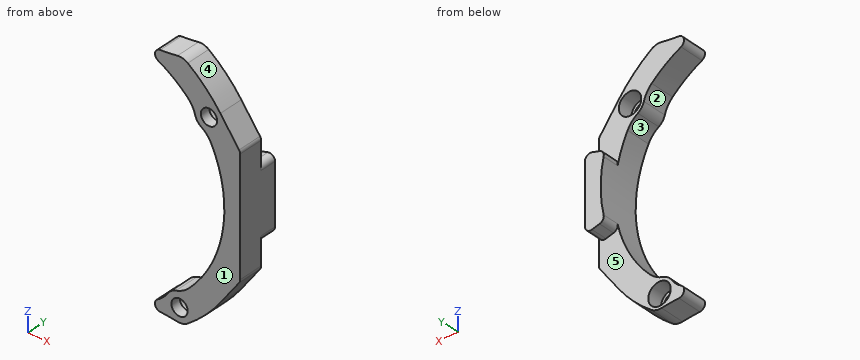
from build123d import *

# Parameters (mm, degrees)
SKETCH_1_R                     = 1.0250000000000292
EXTRUDE_1_DEPTH                = 4.5
EXTRUDE_1_2_DEPTH              = 4.5
EXTRUDE_START                  = -4.5
EXTRUDE_2_DEPTH                = 4.5
EXTRUDE_3_DEPTH                = 3
SKETCH_7_R                     = 1.45
SKETCH_7_R_2                   = 1.0000000000000018
EXTRUDE_5_DEPTH                = 4.5
HOLE_WIZARD_M2_5_2_D           = 2.9
HOLE_WIZARD_M2_5_2_CBORE_D     = 4
HOLE_WIZARD_M2_5_2_CBORE_DEPTH = 2.7
FILLET_5_R                     = 1


with BuildPart() as part:
    # Sketch 1 → Extrude 1 (new body)
    with BuildSketch(Plane(origin=(0, 0, 0), x_dir=(1, 0, 0), z_dir=(0, 1, 0))):
        with BuildLine():
            ThreePointArc((21.348606100588817, 5.102893058050916), (21.291819851832585, 9.358175160870491), (21.68743992704855, 13.595407182923395))
            ThreePointArc((21.687439927048548, 13.595407182923395), (21.641903090720017, 14.556584323583055), (21.236696102342364, 15.429362872677498))
            ThreePointArc((21.236696102342368, 15.429362872677501), (18.56155300614698, 18.56155300614684), (15.429362872677654, 21.236696102342243))
            ThreePointArc((15.429362872677654, 21.23669610234224), (14.556584323583243, 21.641903090720017), (13.595407182923555, 21.68743992704845))
            ThreePointArc((13.595407182923555, 21.687439927048445), (10.687287616312432, 21.367018761558228), (7.763526238556964, 21.26002089734574))
            ThreePointArc((7.763526238556963, 21.260020897345733), (6.432472496268358, 21.282173332286177), (5.102893058051164, 21.348606100588782))
            ThreePointArc((5.1028930580511656, 21.348606100588796), (7.485262352646101, 20.634276035569133), (9.771526987407864, 19.65501870602934))
            ThreePointArc((9.771526987407862, 19.655018706029338), (10.918636162855368, 18.878721056795385), (11.820114941555765, 17.82713486814756))
            ThreePointArc((11.820114941555765, 17.82713486814756), (12.461047348600456, 17.151160280748954), (13.301996390818283, 16.750484973796134))
            ThreePointArc((13.301996390818283, 16.750484973796134), (14.580686550664556, 16.218085710353485), (15.673465718169814, 15.367009220448802))
            ThreePointArc((15.673465718169815, 15.367009220448805), (19.20928084513133, 10.621018285120913), (21.348606100588796, 5.102893058050913))
        make_face()
        with Locations(Location((13.959899741946257, 19.214153616405042, 0), (0, 0, 270))):
            Circle(SKETCH_1_R, mode=Mode.SUBTRACT)
    extrude(amount=EXTRUDE_1_DEPTH)



with BuildPart() as body_2:
    # Sketch 1 → Extrude 1 2 (new body)
    with BuildSketch(Plane(origin=(0, 0, 0), x_dir=(1, 0, 0), z_dir=(0, 1, 0))):
        with BuildLine():
            ThreePointArc((21.687439927048345, -13.59540718292358), (21.291819851832443, -9.358175160870594), (21.348606100588746, -5.102893058050941))
            ThreePointArc((21.348606100588746, -5.10289305805094), (20.63427603556909, -7.4852623526459166), (19.655018706029292, -9.771526987407722))
            ThreePointArc((19.655018706029292, -9.77152698740772), (18.87872105679534, -10.918636162855227), (17.827134868147517, -11.82011494155563))
            ThreePointArc((17.827134868147517, -11.82011494155563), (17.151160280748865, -12.461047348600282), (16.7504849737961, -13.301996390818143))
            ThreePointArc((16.7504849737961, -13.301996390818143), (16.218085710353446, -14.580686550664424), (15.367009220448757, -15.673465718169691))
            ThreePointArc((15.367009220448761, -15.673465718169693), (10.621018285120737, -19.209280845131296), (5.1028930580505785, -21.348606100588768))
            ThreePointArc((5.102893058050578, -21.348606100588754), (9.35817516087026, -21.29181985183253), (13.595407182923264, -21.68743992704851))
            ThreePointArc((13.595407182923264, -21.687439927048516), (13.777164655836453, -21.707466249891656), (13.959899741946161, -21.714153616404968))
            ThreePointArc((13.959899741946161, -21.714153616404968), (14.732442227883533, -21.591794907142855), (15.429362872677345, -21.236696102342332))
            ThreePointArc((15.429362872677347, -21.236696102342336), (18.561553006146696, -18.561553006146962), (21.23669610234214, -15.429362872677675))
            ThreePointArc((21.236696102342137, -15.429362872677672), (21.64190309071992, -14.556584323583264), (21.687439927048352, -13.595407182923577))
        make_face()
        with BuildLine():
            ThreePointArc((19.21415361640496, -12.509899741946258), (20.66415361640495, -13.95989974194627), (19.214153616404936, -15.409899741946257))
            ThreePointArc((19.214153616404936, -15.409899741946255), (17.76415361640495, -13.959899741946243), (19.21415361640496, -12.509899741946256))
        make_face(mode=Mode.SUBTRACT)
    extrude(amount=EXTRUDE_1_2_DEPTH)


with BuildPart() as part_1:
    add(part.part)

    add(body_2.part)  # Extrude 2 merges body 2
    # Sketch 4 → Extrude 2 (add)
    with BuildSketch(Plane(origin=(0, 4.5, 0), x_dir=(1, 0, 0), z_dir=(0, 1, 0)).offset(EXTRUDE_START)):
        with BuildLine():
            Line((21.236696102342133, -15.429362872677666), (24.7634076160975, -10.575260906428365))
            Line((24.7634076160975, -10.575260906428365), (24.7634076160975, 10.575260906428364))
            Line((24.7634076160975, 10.575260906428364), (21.236696102342353, 15.429362872677489))
            ThreePointArc((21.236696102342353, 15.429362872677489), (21.641903090720028, 14.556584323583055), (21.687439927048562, 13.595407182923394))
            ThreePointArc((21.687439927048562, 13.595407182923394), (21.2918198518326, 9.358175160870505), (21.348606100588814, 5.102893058050923))
            ThreePointArc((21.348606100588814, 5.102893058050923), (21.950000000000014, -1.41e-14), (21.34860610058875, -5.102893058050941))
            ThreePointArc((21.34860610058875, -5.102893058050941), (21.291819851832443, -9.358175160870587), (21.687439927048448, -13.595407182923562))
            ThreePointArc((21.687439927048448, -13.595407182923562), (21.64190309071992, -14.556584323583241), (21.236696102342133, -15.429362872677666))
        make_face()
    extrude(amount=EXTRUDE_2_DEPTH)

    # Sketch 5 → Extrude 3 (add)
    with BuildSketch(Plane(origin=(0, 4.5, 0), x_dir=(1, 0, 0), z_dir=(0, 1, 0))):
        with BuildLine():
            Line((21.20207188704507, -5.68107804000035), (24.7634076160975, -6.635335072576056))
            Line((24.7634076160975, -6.635335072576056), (24.7634076160975, 6.635335072576056))
            Line((24.7634076160975, 6.635335072576056), (21.202071887045097, 5.681078040000357))
            ThreePointArc((21.202071887045097, 5.681078040000357), (21.950000000000045, 2.96e-15), (21.20207188704507, -5.68107804000035))
        make_face()
    extrude(amount=EXTRUDE_3_DEPTH)

    # Sketch 7 → Extrude 5 (add)
    with BuildSketch(Plane(origin=(0, 4.5, 0), x_dir=(1, 0, 0), z_dir=(0, 1, 0)).offset(EXTRUDE_START)):
        with Locations((19.21415361640495, -13.959899741946257)):
            Circle(SKETCH_7_R)
        with Locations(Location((19.21415361640495, -13.959899741946257, 0), (0, 0, 270))):
            Circle(SKETCH_7_R_2, mode=Mode.SUBTRACT)
    extrude(amount=EXTRUDE_5_DEPTH)

    # Hole Wizard M2.5 _2 (through all)
    with Locations(Plane(origin=(13.959899742, 4.5, -19.214153616), x_dir=(0, 0, 1), z_dir=(0, 1, 0))):
        with Locations((0, 0), (33.174053358, 5.254253874)):
            CounterBoreHole(HOLE_WIZARD_M2_5_2_D / 2, HOLE_WIZARD_M2_5_2_CBORE_D / 2, HOLE_WIZARD_M2_5_2_CBORE_DEPTH)

    # Fillet 5
    fillet_5_edges = [part_1.edges().sort_by_distance(p)[0] for p in [
        (24.7634076160975, 2.25, 10.575260906428365),
        (24.7634076160975, 2.25, -10.575260906428364),
        (24.7634076160975, 6, -6.635335072576056),
        (21.202071887045093, 6, -5.681078040000356),
        (21.202071887045065, 6, 5.681078040000351),
        (24.7634076160975, 6, 6.635335072576056),
        (5.1028930580505785, 2.25, 21.34860610058876),
        (5.102893058051165, 2.25, -21.34860610058879),
    ]]
    fillet(fillet_5_edges, radius=FILLET_5_R)


solid = part_1.part
Geometry check sheet. Reference: the model listing, model coordinates, mm. Face numbers are marked on the shaded views. A direction names the side the tool comes from. Give positions to 0.01 mm unless a question says otherwise; leave off trailing zeros. Loops run counter-clockwise (first coordinate to the right, second up) from the corner with the lowest first, then second, coordinate; pieces in that order, holes last. Notation, with made-up numbers: M -37,15 L -33,15 A21 ccw -33,22 Z; hole C 10,34 d6. An arc over 180 degrees is marked long. Answer as a JSON object with one key per item and string values. Group by question number.
Item 1: Sectioned sample at D-D on y = 2.75. Give the number of separate pieces and of enclosed holes in the cut face, plus the area to 3 significant figures.
Item 2: Sectioned sample at C-C on z = -1. Record the boundary of the cut face in (x, y), plus the area to 3 significant figures.
Item 3: Sectioned sample at B-B on x = 23. Record the boundary of the cut face in (y, z).
Item 4: Sectioned sample at A-A on y = 5. Record the boundary of the cut face in (x, z).
Item 5: Access from +Z, -Z, +X, -X, +Y, -Y to the whole of each face (thin tool, end or side, straight path). Record for the marked faces 1 and 2.
Item 6: Material ranges on L1, parallel to Z at x = 19.5, y = 3; L2, parallel to Z at x = 15.25, y = 1; L3, parallel to X at y = 4.75, z = 5, recorded low to high.
Item 7: Mould release check, pull along Z, two halves, no side actions. Record for the marked faces 3, 4 and 5: pulls with the +Z half, pulls with the -Z half, needs draft (parallel to the pull), parting line crosses it, or undercut.
Item 8: Gauge pin test, flat ends, axial feed: pin 1 (8 mm diameter, centred on x = 17, z = -17, fed in from -Y); pin 2 (5 mm diameter, centred on x = 13.96, z = -19.21, fed in from +Y); pin 3 (3 mm diameter, centred on x = 20.5, y = 4.5, fed in from -Z). Record the tip position at first contact, or that the pin passes through.
Findings below:
{
 "1": {"separate pieces": "1", "enclosed holes": "2", "area": "189 mm2"},
 "2": {"outline": "M 21.93,0 L 24.76,0 L 24.76,7.5 L 21.93,7.5 Z", "area": "21.3 mm2"},
 "3": {"outline": "M 0,-13 L 4.5,-13 L 4.5,-6.16 L 7.5,-6.16 L 7.5,6.16 L 4.5,6.16 L 4.5,13 L 0,13 Z"},
 "4": {"outline": "M 21.43,-4.75 A1 ccw 22.15,-5.93 L 23.5,-6.3 A1 ccw 24.76,-5.33 L 24.76,5.33 A1 ccw 23.5,6.3 L 22.15,5.93 A1 ccw 21.43,4.75 A21.95 cw Z"},
 "5": {"face 1": "+Z, -Z, +X, -X, -Y", "face 2": "-X, +Y, -Y"},
 "6": {"L1": "-17.57 to -10.08, 10.06 to 11.98, 15.94 to 17.57", "L2": "-21.36 to -19.88, -18.55 to -15.75, 15.79 to 21.36", "L3": "21.41 to 24.76"},
 "7": {"face 3": "undercut", "face 4": "pulls with the +Z half", "face 5": "needs draft"},
 "8": {"pin 1": "y = 0", "pin 2": "y = 4.5", "pin 3": "z = -18.11"}
}
